from build123d import *

# Parameters (mm, degrees)
BOSS_EXTRUDE1_DEPTH = 155
SKETCH4_W           = 144
SKETCH4_H           = 111
CUT_EXTRUDE1_DEPTH  = 5
SKETCH5_R           = 38.5
CUT_EXTRUDE2_DEPTH  = 10
BOSS_EXTRUDE2_DEPTH = 5
CUT_EXTRUDE3_DEPTH  = 5
CUT_EXTRUDE4_DEPTH  = 2.5
CUT_EXTRUDE5_DEPTH  = 2.5
BOSS_EXTRUDE3_DEPTH = 142
SKETCH12_R          = 38.5
CUT_EXTRUDE6_DEPTH  = 6.5
BOSS_EXTRUDE4_DEPTH = 147
CUT_EXTRUDE7_DEPTH  = 25
SKETCH16_R          = 1.5
CUT_EXTRUDE8_DEPTH  = 5
SKETCH17_R          = 1.5875
CUT_EXTRUDE9_DEPTH  = 10


with BuildPart() as part:
    # Sketch3 → Boss-Extrude1 (new body)
    with BuildSketch(Plane(origin=(0, 0, 0), x_dir=(0, 0, -1), z_dir=(1, 0, 0))):
        Polygon((58.381197846, 114.119200877), (0.860471904, 14.490381057), (12.979274058, -6.5), (132.75, -6.5), (142.504165125, 10.394709581), (82.618802154, 114.119200877), align=None)
        Polygon((7.5, 12.990381057), (15, 0), (15, -1.5), (126, -1.5), (126, 0), (133.5, 12.990381057), (134.799038106, 13.740381057), (79.299038106, 109.869200877), (78, 109.119200877), (63, 109.119200877), (61.700961894, 109.869200877), (6.200961894, 13.740381057), align=None, mode=Mode.SUBTRACT)
    extrude(amount=BOSS_EXTRUDE1_DEPTH)

    # Sketch4 → Cut-Extrude1 (cut)
    with BuildSketch(Plane(origin=(0, 3.25, 5.629165125), x_dir=(1, 0, 0), z_dir=(0, 0.4999999999999995, 0.8660254037844389))):
        with Locations((77.5, 70.5)):
            Rectangle(SKETCH4_W, SKETCH4_H)
    extrude(amount=-CUT_EXTRUDE1_DEPTH, mode=Mode.SUBTRACT)

    # Sketch5 → Cut-Extrude2 (cut)
    with BuildSketch(Plane(origin=(0, 64.304790967, -111.379165125), x_dir=(-1, 0, 0), z_dir=(0, 0.5000000000000006, -0.8660254037844385))):
        with Locations(Location((-77.5, -2.364637029, 0), (0, 0, 90))):
            Circle(SKETCH5_R)
    extrude(amount=-CUT_EXTRUDE2_DEPTH, mode=Mode.SUBTRACT)


with BuildPart() as body_2:
    # Sketch6 → Boss-Extrude2 (new body)
    with BuildSketch(Plane(origin=(155, 0, 0), x_dir=(0, 0, -1), z_dir=(1, 0, 0))):
        Polygon((82.618802154, 114.119200877), (58.381197846, 114.119200877), (0.860471904, 14.490381057), (12.979274058, -6.5), (132.75, -6.5), (142.504165125, 10.394709581), align=None)
    extrude(amount=BOSS_EXTRUDE2_DEPTH)

    # Sketch7 → Cut-Extrude3 (cut)
    with BuildSketch(Plane(origin=(160, 0, 0), x_dir=(0, 0, -1), z_dir=(1, 0, 0))):
        Polygon((63, 109.119200877), (7.5, 12.990381057), (15, 0), (126, 0), (133.5, 12.990381057), (78, 109.119200877), align=None)
    extrude(amount=-CUT_EXTRUDE3_DEPTH, mode=Mode.SUBTRACT)

    # Sketch8 → Cut-Extrude4 (cut)
    with BuildSketch(Plane(origin=(160, 0, 0), x_dir=(0, 0, -1), z_dir=(1, 0, 0))):
        Polygon((6.200961894, 13.740381057), (61.700961894, 109.869200877), (59.968911087, 110.869200877), (4.468911087, 14.740381057), align=None)
    extrude(amount=-CUT_EXTRUDE4_DEPTH, mode=Mode.SUBTRACT)

    # Sketch10 → Cut-Extrude5 (cut)
    with BuildSketch(Plane(origin=(160, 0, 0), x_dir=(0, 0, -1), z_dir=(1, 0, 0))):
        Polygon((42.75, 74.045172024), (27.75, 48.06440991), (26.450961894, 48.81440991), (41.450961894, 74.795172024), align=None)
    extrude(amount=-CUT_EXTRUDE5_DEPTH, mode=Mode.SUBTRACT)

    # Sketch11 → Boss-Extrude3 (add)
    with BuildSketch(Plane(origin=(160, 0, 0), x_dir=(0, 0, -1), z_dir=(1, 0, 0))):
        Polygon((63, 109.119200877), (62, 107.387150069), (60.700961894, 108.137150069), (61.700961894, 109.869200877), (59.968911087, 110.869200877), (58.968911087, 109.137150069), (56.370834875, 110.637150069), (58.381197846, 114.119200877), (82.618802154, 114.119200877), (142.504165125, 10.394709581), (132.75, -6.5), (12.979274058, -6.5), (0.860471904, 14.490381057), (2.870834875, 17.972431864), (5.468911087, 16.472431864), (4.468911087, 14.740381057), (6.200961894, 13.740381057), (7.200961894, 15.472431864), (8.5, 14.722431864), (7.5, 12.990381057), (15, 0), (126, 0), (133.5, 12.990381057), (78, 109.119200877), align=None)
    extrude(amount=BOSS_EXTRUDE3_DEPTH)

    # Sketch12 → Cut-Extrude6 (cut)
    with BuildSketch(Plane(origin=(0, 64.304790967, -111.379165125), x_dir=(-1, 0, 0), z_dir=(0, 0.5000000000000006, -0.8660254037844384))):
        with Locations(Location((-232.5, -2.364637029, 0), (0, 0, 90))):
            Circle(SKETCH12_R)
    extrude(amount=-CUT_EXTRUDE6_DEPTH, mode=Mode.SUBTRACT)

    # Sketch13 → Boss-Extrude4 (add)
    with BuildSketch(Plane.ZY.offset(-155)):
        Polygon((-26.593395609, 30.661112341), (-21.593395609, 22.000858303), (-14.925, 25.850858303), (-13.925, 24.118807495), (-20.593395609, 20.268807495), (-11.945597073, 5.290381057), (-13.100297611, 3.290381057), (-28.325446417, 29.661112341), align=None)
        Polygon((-62.243395609, 92.408723631), (-55.575, 96.258723631), (-56.575, 97.990774438), (-63.243395609, 94.140774438), (-71.891194146, 109.119200877), (-74.200595222, 109.119200877), (-58.975446417, 82.748469593), (-57.243395609, 83.748469593), align=None)
    extrude(amount=-BOSS_EXTRUDE4_DEPTH)

    # Sketch14 → Cut-Extrude7 (cut)
    with BuildSketch(Plane.XY.offset(-150)):
        with BuildLine():
            Line((234.6666, 5.5875), (226.437, 5.5875))
            ThreePointArc((226.437, 5.5875), (226.167592316, 5.699092316), (226.056, 5.9685))
            Line((226.056, 5.9685), (226.056, 12.0391))
            ThreePointArc((226.056, 12.0391), (230.5518, 16.5349), (235.0476, 12.0391))
            Line((235.0476, 12.0391), (235.0476, 5.9685))
            ThreePointArc((235.0476, 5.9685), (234.936007684, 5.699092316), (234.6666, 5.5875))
        make_face()
        with BuildLine():
            Line((265.299934, 6.0875), (255.899934, 6.0875))
            ThreePointArc((255.899934, 6.0875), (255.192827219, 6.380393219), (254.899934, 7.0875))
            Line((254.899934, 7.0875), (254.899934, 15.5875))
            ThreePointArc((254.899934, 15.5875), (255.192827219, 16.294606781), (255.899934, 16.5875))
            Line((255.899934, 16.5875), (265.299934, 16.5875))
            ThreePointArc((265.299934, 16.5875), (266.007040781, 16.294606781), (266.299934, 15.5875))
            Line((266.299934, 15.5875), (266.299934, 7.0875))
            ThreePointArc((266.299934, 7.0875), (266.007040781, 6.380393219), (265.299934, 6.0875))
        make_face()
    extrude(amount=CUT_EXTRUDE7_DEPTH, mode=Mode.SUBTRACT)

    # Sketch16 → Cut-Extrude8 (cut)
    with BuildSketch(Plane(origin=(0, -4.85, -8.400446417), x_dir=(-1, 0, 0), z_dir=(0, -0.4999999999999997, -0.8660254037844389))):
        with Locations(Location((-172.60681079, 106.05, 0), (0, 0, 90))):
            Circle(SKETCH16_R)
        with Locations(Location((-172.60681079, 34.95, 0), (0, 0, 90))):
            Circle(SKETCH16_R)
        with Locations(Location((-290.71681079, 106.05, 0), (0, 0, 90))):
            Circle(SKETCH16_R)
        with Locations(Location((-290.71681079, 34.95, 0), (0, 0, 90))):
            Circle(SKETCH16_R)
    extrude(amount=-CUT_EXTRUDE8_DEPTH, mode=Mode.SUBTRACT)

    # Sketch17 → Cut-Extrude9 (cut)
    with BuildSketch(Plane(origin=(0, 0, 0), x_dir=(1, 0, 0), z_dir=(0, 1, 0))):
        with Locations(Location((230.12, 51.9601016, 0), (0, 0, 270))):
            Circle(SKETCH17_R)
        with Locations(Location((258.06, 51.9601016, 0), (0, 0, 270))):
            Circle(SKETCH17_R)
        with Locations(Location((273.3, 102.7601016, 0), (0, 0, 270))):
            Circle(SKETCH17_R)
    extrude(amount=-CUT_EXTRUDE9_DEPTH, mode=Mode.SUBTRACT)


solid = body_2.part
The model under review builds one solid part; all positions refer to its coordinate system, in mm. A direction names the side the tool comes from. Coordinates: 2 decimals unless noted, no trailing zeros. Write each loop counter-clockwise with the first axis right and the second up, starting at its lowest first coordinate (ties: lowest second). Pieces come first, ordered by that corner, then holes. Notation, with made-up numbers: (45.25, 63) -> (81.25, 63) arc R20 cw to (81.25, 88) -> close; hole circle Ø1 at (78.25, 13). An arc over 180 degrees is marked (long way). Answer in a Markdown table with one row per item.
1. We need section B-B, the plane z = -124. Give the number of separate pieces and of enclosed holes in the cut face, and give its area (3 significant figures).
Answers below:
| item | result |
|---|---|
| separate pieces | 3 |
| enclosed holes | 0 |
| area | 2,210 mm^2 |
2. For faces 1 (the flat face through (194.804, 71.063, -99.972)), 2 (the flat face through (254.9, 11, -136)), 3 (the flat face through (155, 63, -35)), list the 3-axis set-ups (+Z, -Z, +X, -X, +Y, -Y) from which the entire face can be reached by the end or side of a thin tool; tool diameter is ignored.
Answers below:
| item | result |
|---|---|
| face 1 | +X, -X |
| face 2 | -Z |
| face 3 | +Z, -Z, -X, +Y, -Y |
3. We need section A-A, the plane z = -85. State the section outline as (x, y) points.
Answers below:
| item | result |
|---|---|
| outline | (155, -6.5) -> (302, -6.5) -> (302, 0) -> (155, 0) -> close; (155, 96.99) -> (302, 96.99) -> (302, 109.99) -> (155, 109.99) -> close |
4. Clearance check with flat-ended pins moving along their axes: pin 1 Ø2 at (x, z) = (264.5, -32.5) entering from +Y; pin 2 Ø1.9 at (x, z) = (273.3, -102.76) entering from +Y; pin 3 Ø1 at (x, z) = (252.5, -93) entering from +Y. State where each tip first meets the part, or that it passes through.
Answers below:
| item | result |
|---|---|
| pin 1 | stops at y = 0 |
| pin 2 | stops at y = 80.88 |
| pin 3 | stops at y = 97 |
5. Wall thickness on probe 1 along Y at (x, z) = (179, -35.5); probe 2 along Z at (x, y) = (230, -4); probe 3 along Y at (x, z) = (200, -122): over which ranges is each line inside the solid? List them lowest first. Write a range as [from, to].
Answers below:
| item | result |
|---|---|
| probe 1 | y = [-6.5, 0] |
| probe 2 | z = [-134.19, -53.54], [-50.38, -11.54] |
| probe 3 | y = [-6.5, 0], [32.91, 43.87] |
6. Draft analysis for pull direction Z (two halves, no side actions). For faces 4 (the flat face through (156.979, 61.548, -35.535)), 5 (the flat face through (227.47, 2.07, -137.7)), 6 (the flat face through (160, 91, -52)), state which applies: +Z half, -Z half, draft (parallel to the pull), parting line (faces both ways), or undercut.
Answers below:
| item | result |
|---|---|
| face 4 | undercut |
| face 5 | -Z half |
| face 6 | draft |
